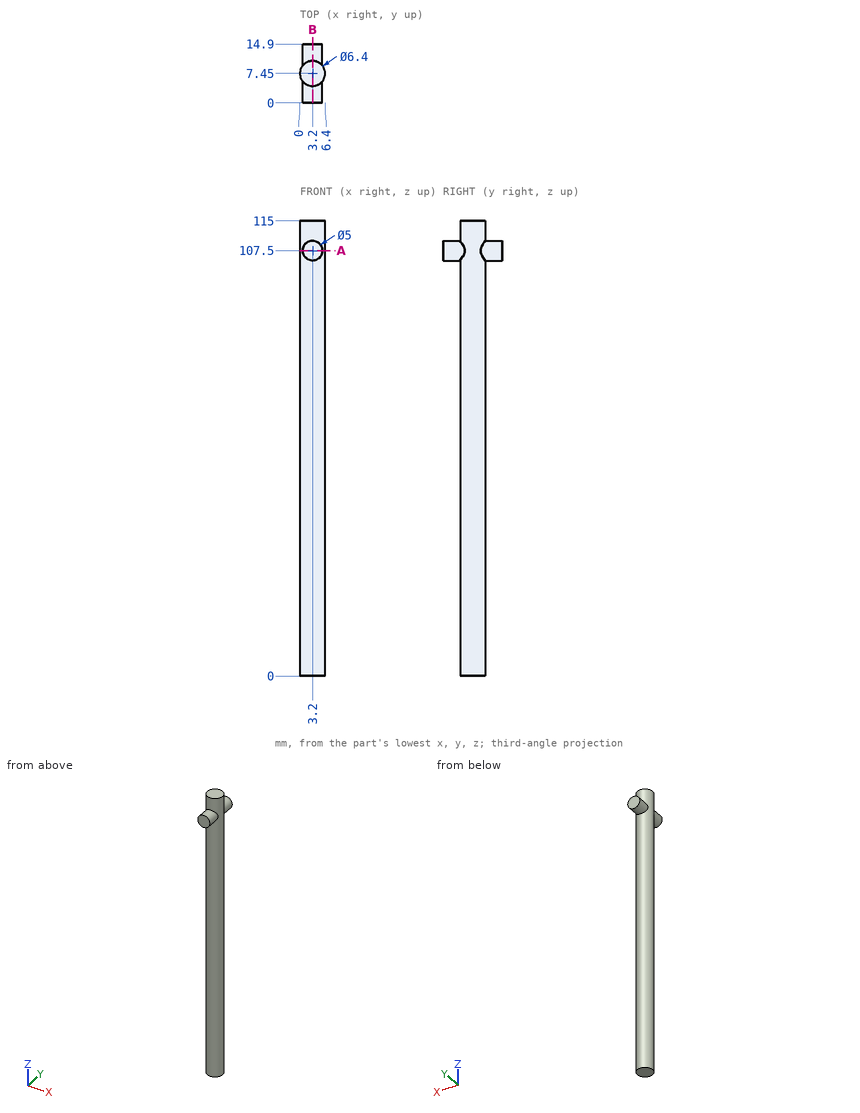
Geometry check sheet. Reference: drawing and pictorial views, mm from the part's lowest x, y, z. Coordinates: 2 decimals unless noted, no trailing zeros. Order: outer loops, then holes, each group sorted by start corner. A loop starts at its lowest first (then second) coordinate and runs counter-clockwise, first axis right, second up.
Item 1: Section check A-A (z = 107.5). Enter the section's corners in (x, y), plus the area to 3 significant figures.
Item 2: Section check B-B (x = 3.2). Enter the section's corners in (y, z).
Item 3: Scan lines: line 1 along Z through (x, y) = (3.5, 13.25); line 2 along Y through (x, z) = (3.5, 7); line 3 along X through (y, z) = (7.75, 56.5). Record each from-to range of solid material in increasing order.
Item 4: Depth check by flat-ended pin: pin 1 (2 mm diameter, centred on x = 3, z = 74, fed in from +Y). Enter the tip coordinate at first touch or a pass-through.
Check sheet entries:
1. outline: (0.7, 0) - (5.7, 0) - (5.7, 5.45) arc R3.2 ccw to (5.7, 9.45) - (5.7, 14.9) - (0.7, 14.9) - (0.7, 9.45) arc R3.2 ccw to (0.7, 5.45) - close
1. area: 78.3 mm2
2. outline: (0, 105) - (4.25, 105) - (4.25, 0) - (10.65, 0) - (10.65, 105) - (14.9, 105) - (14.9, 110) - (10.65, 110) - (10.65, 115) - (4.25, 115) - (4.25, 110) - (0, 110) - close
3. line 1: z = 105.02 to 109.98
3. line 2: y = 4.26 to 10.64
3. line 3: x = 0.01 to 6.39
4. pin 1: stops at y = 10.65
